The drawing under review shows one solid part. Ordinate dimensions are in mm from its lowest x, y, z. A direction names the side the tool comes from. Coordinates: 2 decimals unless noted, no trailing zeros. Loops run counter-clockwise (first coordinate to the right, second up) from the corner with the lowest first, then second, coordinate; pieces in that order, holes last. Notation, with made-up numbers: M 79,45 L 101,45 A23 ccw 101,65 Z; hole C -16.75,66.5 d2. An arc over 180 degrees is marked long. Return JSON: item names as keys, results as strings.
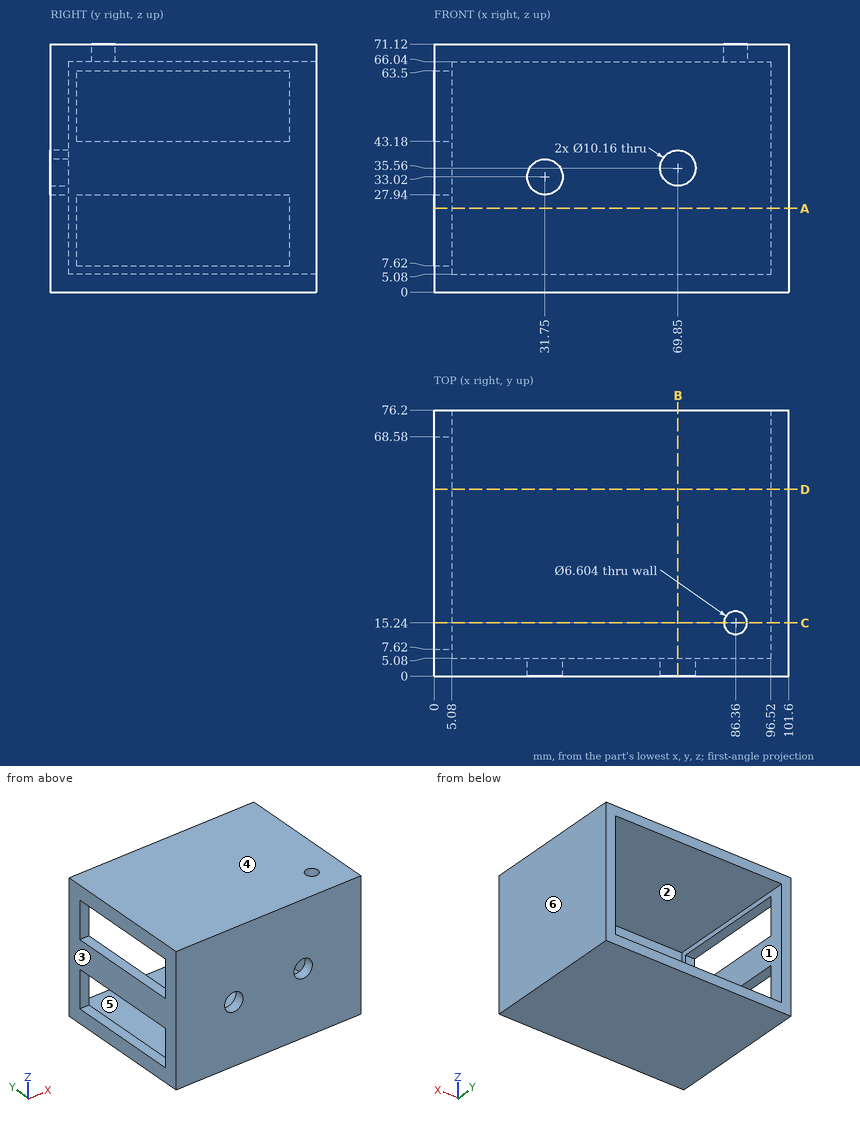
1. The part is to be moulded in two halves that separate along Z. For the marked faces 1, 2, 3 and 4, say which applies: released by +Z, released by -Z, zero draft, split by the parting line, or undercut.
Check values:
{"face 1": "undercut", "face 2": "undercut", "face 3": "zero draft", "face 4": "released by +Z"}
2. Insertion check: pin 1 Ø5 at (x, z) = (41, 37.5) entering from +Y; pin 2 Ø4 at (y, z) = (50, 52.5) entering from -X; pin 3 Ø9 at (x, z) = (69.85, 35.56) entering from +Y. Each pin has a flat end and moves straight along its axis. Give the tip position at first contact, or say it passes through.
Check values:
{"pin 1": "y = 5.08", "pin 2": "x = 96.52", "pin 3": "through"}
3. To check wall thickness, follow line 1 (Z direction, x = 48, y = 57); line 2 (X direction, y = 15, z = 68); line 3 (X direction, y = 69, z = 29). State the ranges of each line that lie inside material, in increasing order.
Check values:
{"line 1": "0 to 5.08, 66.04 to 71.12", "line 2": "0 to 83.07, 89.65 to 101.6", "line 3": "0 to 5.08, 96.52 to 101.6"}
4. Add section D-D on y = 53.5. Give the boundary of the cut face in (x, z).
Check values:
{"outline": "M 0,0 L 101.6,0 L 101.6,71.12 L 0,71.12 L 0,63.5 L 5.08,63.5 L 5.08,66.04 L 96.52,66.04 L 96.52,5.08 L 5.08,5.08 L 5.08,7.62 L 0,7.62 Z; M 0,27.94 L 5.08,27.94 L 5.08,43.18 L 0,43.18 Z"}
5. Add section C-C on y = 15.24. Give the boundary of the cut face in (x, z), plus the area to 3 significant figures.
Check values:
{"outline": "M 0,0 L 101.6,0 L 101.6,71.12 L 89.66,71.12 L 89.66,66.04 L 96.52,66.04 L 96.52,5.08 L 5.08,5.08 L 5.08,7.62 L 0,7.62 Z; M 0,27.94 L 5.08,27.94 L 5.08,43.18 L 0,43.18 Z; M 0,63.5 L 5.08,63.5 L 5.08,66.04 L 83.06,66.04 L 83.06,71.12 L 0,71.12 Z", "area": "1,410 mm²"}
6. Machinability: for the marked faces 5 and 6, which of the approach directions +Z, -Z, +X, -X, +Y, -Y give a long, thin tool a straight path to every point of the face, cutting with its end or side? Answer none if there is none.
Check values:
{"face 5": "+Y", "face 6": "+Z, -Z, +X, +Y, -Y"}
7. Add section A-A on z = 24. Give the boundary of the cut face in (x, y).
Check values:
{"outline": "M 0,0 L 101.6,0 L 101.6,76.2 L 96.52,76.2 L 96.52,5.08 L 5.08,5.08 L 5.08,7.62 L 0,7.62 Z; M 0,68.58 L 5.08,68.58 L 5.08,76.2 L 0,76.2 Z"}
8. Add section B-B on x = 69.85. Give the boundary of the cut face in (y, z), plus the area to 3 significant figures.
Check values:
{"outline": "M 0,0 L 76.2,0 L 76.2,5.08 L 5.08,5.08 L 5.08,30.48 L 0,30.48 Z; M 0,40.64 L 5.08,40.64 L 5.08,66.04 L 76.2,66.04 L 76.2,71.12 L 0,71.12 Z", "area": "1,030 mm²"}
